Verification items for the finished model (mm, model axes). A direction names the side the tool comes from. Give positions to 0.01 mm unless a question says otherwise; leave off trailing zeros. Loops run counter-clockwise (first coordinate to the right, second up) from the corner with the lowest first, then second, coordinate; pieces in that order, holes last. Notation, with made-up numbers: M 73.25,53 L 111.25,53 A23 cw 111.25,63 Z; hole C 59,19.25 d10. An arc over 180 degrees is marked long. Use a Markdown table: item, result.
from build123d import *

# Parameters (mm, degrees)
F3_W      = 5.08
F3_H      = 12.7
F6_W      = 55.88
F6_H      = 20.32
F7_DEPTH  = 6.35
F10_W     = 5.08
F10_H     = 12.7
F12_W     = 55.88
F12_H     = 20.32
F13_DEPTH = 6.35
F14_R     = 5.08
F15_R     = 5.08
F16_R     = 5.07999


# Not quite as in the source:
# - a fillet or chamfer is up to 0.001 mm smaller than in the source, because OpenCascade refuses the exact size


with BuildPart() as f1:
    # F0 (on Right) → F1 (revolve)
    with BuildSketch(Plane.YZ):
        with BuildLine():
            Line((63.5, 5.08), (0, 5.08))
            Line((0, 5.08), (0, 0))
            Line((0, 0), (63.3201003075, 0))
            ThreePointArc((63.3201003075, 0), (67.2357467781, 1.5686265864), (68.58, 5.5668586865))
            Line((68.58, 5.5668586865), (68.58, 148.1529325247))
            ThreePointArc((68.58, 148.1529325247), (70.7035337377, 150.2764662623), (68.58, 152.4))
            Line((68.58, 152.4), (63.5, 152.4))
            Line((63.5, 152.4), (63.5, 5.08))
        make_face()
    revolve(axis=Axis((0, 0, 2.54), (0, 0, 1)))

    # F3 (on offset) → F4 (join, up to the next surface of F1)
    with BuildSketch(Plane.XZ.offset(86.36)):
        with Locations((-20.32, 125.8009325247)):
            Rectangle(F3_W, F3_H)
        with Locations((20.32, 125.8009325247)):
            Rectangle(F3_W, F3_H)
    extrude(until=Until.NEXT, dir=(0, 1, 0))

    # F6 (on offset) → F7 (join, through all)
    with BuildSketch(Plane.XZ.offset(92.71)):
        with Locations((0, 129.1029325247)):
            Rectangle(F6_W, F6_H)
    extrude(amount=-F7_DEPTH)

    # F10 (on offset) → F11 (join, up to the next surface of F1)
    with BuildSketch(Plane.XZ.offset(-86.36)):
        with Locations((20.32, 125.8009325247)):
            Rectangle(F10_W, F10_H)
        with Locations((-20.32, 125.8009325247)):
            Rectangle(F10_W, F10_H)
    extrude(until=Until.NEXT)

    # F12 (on offset) → F13 (join, through all)
    with BuildSketch(Plane.XZ.offset(-92.71)):
        with Locations((0, 129.1029325247)):
            Rectangle(F12_W, F12_H)
    extrude(amount=F13_DEPTH)

    # F14
    f14_edges = [f1.edges().sort_by_distance(p)[0] for p in [
        (0, -92.71, 118.942933),
    ]]
    fillet(f14_edges, radius=F14_R)

    # F15
    f15_edges = [f1.edges().sort_by_distance(p)[0] for p in [
        (0, 92.71, 118.942933),
    ]]
    fillet(f15_edges, radius=F15_R)

    # F16 (radius 5.08 in the source; OpenCascade refuses exactly that, so slightly less here)
    f16_edges = [f1.edges().sort_by_distance(p)[0] for p in [
        (-22.86, 75.508922, 119.450933),
        (22.86, 75.508922, 119.450933),
        (-22.86, -75.508922, 119.450933),
        (22.86, -75.508922, 119.450933),
    ]]
    fillet(f16_edges, radius=F16_R)


solid = f1.part
(1) Set-up check for faces 4 (the cylindrical face through (21.33, 75.36, 120.9)), 5 (the flat face through (-27.94, -90, 129)), 6 (the cylindrical face through (-21.33, 75.36, 120.9)), 7 (the flat face through (-1, -1, 5.08)): record each of +Z, -Z, +X, -X, +Y, -Y from which the full face is reachable in a straight line by a thin tool's end or side.
Results below:
| item | result |
|---|---|
| face 4 | -Z, +X |
| face 5 | +Z, -Z, -X, -Y |
| face 6 | -Z, -X |
| face 7 | +Z |
(2) Gauge pin test, flat ends, axial feed: P1, Ø5, axis at x = -6.5, y = 88, coming from the +Z side; P2, Ø8.5, axis at y = -71.5, z = 130, coming from the +X side; P3, Ø4, axis at x = -19.5, y = -73.5, coming from the +Z side. Record the tip position at first contact, or that the pin passes through.
Results below:
| item | result |
|---|---|
| P1 | z = 139.26 |
| P2 | x = 22.86 |
| P3 | z = 132.15 |
(3) Cross-section at D-D on y = 0. Record the cut outline in (x, z).
Results below:
| item | result |
|---|---|
| outline | M -68.58,5.57 A5.03 ccw -63.32,0 L 63.32,0 A5.03 ccw 68.58,5.57 L 68.58,148.15 A2.12 ccw 68.58,152.4 L 63.5,152.4 L 63.5,5.08 L -63.5,5.08 L -63.5,152.4 L -68.58,152.4 A2.12 ccw -68.58,148.15 Z |
(4) Draft check along Y on faces 1 (the cylindrical face through (0.39, 91.18, 120.39)), 2 (the flat face through (0, 86.36, 129)), 3 (the flat face through (-27.94, 90, 129)). Enter one of: +Y half, -Y half, draft (parallel to the pull), parting line (faces both ways), or undercut.
Results below:
| item | result |
|---|---|
| face 1 | +Y half |
| face 2 | undercut |
| face 3 | draft |
(5) Material ranges on line 1 (Y direction, x = 0, z = 48.5); line 2 (Z direction, x = 29, y = -46), recorded low to high.
Results below:
| item | result |
|---|---|
| line 1 | -68.58 to -63.5, 63.5 to 68.58 |
| line 2 | 0 to 5.08 |
(6) Cross-section at C-C on z = 19. Record the cut outline in (x, y), then the cut area to 3 significant figures.
Results below:
| item | result |
|---|---|
| outline | C 0,0 d137.16; hole C 0,0 d127 |
| area | 2,110 mm^2 |
(7) Cross-section at B-B on x = 0. Record the cut outline in (y, z).
Results below:
| item | result |
|---|---|
| outline | M -92.71,124.02 A5.08 ccw -87.63,118.94 L -86.36,118.94 L -86.36,139.26 L -92.71,139.26 Z; M -68.58,5.57 A5.03 ccw -63.32,0 L 63.32,0 A5.03 ccw 68.58,5.57 L 68.58,148.15 A2.12 ccw 68.58,152.4 L 63.5,152.4 L 63.5,5.08 L -63.5,5.08 L -63.5,152.4 L -68.58,152.4 A2.12 ccw -68.58,148.15 Z; M 86.36,118.94 L 87.63,118.94 A5.08 ccw 92.71,124.02 L 92.71,139.26 L 86.36,139.26 Z |
